Work out the finished part from the listing and answer in its coordinate system (mm). Round coordinates to 2 decimals unless told otherwise and drop trailing zeros. Loops run counter-clockwise (first coordinate to the right, second up) from the corner with the lowest first, then second, coordinate; pieces in that order, holes last. Notation, with made-up numbers: (-31, -18.75) -> (23, -18.75) arc R8 cw to (23, -14.75) -> close; hole circle Ø10 at (43.5, 28.5). An arc over 180 degrees is marked (long way). Use one line per item in the form item = value.
Autodesk Inventor part; units mm, degrees
ref_plane "YZ Plane" through (0, 0, 0) normal (1, 0, 0) x (0, 1, 0)
ref_plane "XZ Plane" through (0, 0, 0) normal (0, 1, 0) x (-1, 0, 0)
ref_plane "XY Plane" through (0, 0, 0) normal (0, 0, 1) x (1, 0, 0)
sketch "Sketch1" plane through (0, 0, 0) normal (0, 0, 1) x (1, 0, 0)
  circle A0 centre (0, 0) radius 10
  dimension "d0" = 20
extrude "Extrusion1" add sketch "Sketch1" along normal blind 5
sketch "Sketch2" plane through (0, 0, 5) normal (0, 0, 1) x (1, 0, 0)
  circle A0 centre (0, 0) radius 8.5
  dimension "d3" = 17
extrude "Extrusion2" add sketch "Sketch2" along normal blind 2.5
sketch "Sketch3" plane through (0, 0, 7.5) normal (0, 0, 1) x (1, 0, 0)
  circle A0 centre (0, 0) radius 9.9761
extrude "Extrusion3" add sketch "Sketch3" along normal blind 20
sketch "Sketch4" plane through (0, 0, 27.5) normal (0, 0, 1) x (1, 0, 0)
  circle A0 centre (0, 0) radius 8.5
extrude "Extrusion4" add sketch "Sketch4" along normal blind 2.5
sketch "Sketch5" plane through (0, 0, 30) normal (0, 0, 1) x (1, 0, 0)
  circle A0 centre (0, 0) radius 9.9761
extrude "Extrusion5" add sketch "Sketch5" along normal blind 5
sketch "Sketch6" plane through (0, 0, 35) normal (0, 0, 1) x (1, 0, 0)
  line L0 (-13.1636, 0) -> (14.8956, 0)
  line L1 (14.8956, 0) -> (14.8956, -10.45)
  line L2 (14.8956, -10.45) -> (-13.1636, -10.45)
  line L3 (-13.1636, -10.45) -> (-13.1636, 0)
  point P0 (0, 0)
extrude "Extrusion6" cut sketch "Sketch6" against normal blind 35
properties part number "Top Pully"
(1) Find section A-A, the plane x = 0. Write down the section's boundary in (y, z).
Completed:
outline = (0, 0) -> (10, 0) -> (10, 5) -> (8.5, 5) -> (8.5, 7.5) -> (9.98, 7.5) -> (9.98, 27.5) -> (8.5, 27.5) -> (8.5, 30) -> (9.98, 30) -> (9.98, 35) -> (0, 35) -> close
(2) Find section D-D, the plane x = -2.25. Write down the section's boundary in (y, z).
Completed:
outline = (0, 0) -> (9.74, 0) -> (9.74, 5) -> (8.2, 5) -> (8.2, 7.5) -> (9.72, 7.5) -> (9.72, 27.5) -> (8.2, 27.5) -> (8.2, 30) -> (9.72, 30) -> (9.72, 35) -> (0, 35) -> close
(3) For a pull along Z with two mould halves and no side action, classify faces 1 (the flat face through (0, 4, 35)), 2 (the cylindrical face through (-0.219, 9.974, 17.36)), 3 (the flat face through (-1, 9, 30)) as +Z half, -Z half, draft (parallel to the pull), parting line (faces both ways), or undercut.
Completed:
face_1 = +Z half
face_2 = draft
face_3 = undercut
(4) Consider L1, parallel to Z at x = 8.5, y = 1.75; L2, parallel to Y at x = 5.25, z = 8; L3, parallel to X at y = 6.25, z = 28. Determine where each line is inside the solid, lowest interval first.
Completed:
L1 = 0 to 5, 7.5 to 27.5, 30 to 35
L2 = 0 to 8.48
L3 = -5.76 to 5.76
(5) Find section B-B, the plane z = 16. Write down the section's boundary in (x, y), then the cut area to 3 significant figures.
Completed:
outline = (-9.98, 0) -> (9.98, 0) arc R9.98 ccw to start
area = 156 mm2
(6) Find section C-C, the plane y = 4. Write down the section's boundary in (x, z), then the cut area to 3 significant figures.
Completed:
outline = (-9.17, 0) -> (9.17, 0) -> (9.17, 5) -> (7.5, 5) -> (7.5, 7.5) -> (9.14, 7.5) -> (9.14, 27.5) -> (7.5, 27.5) -> (7.5, 30) -> (9.14, 30) -> (9.14, 35) -> (-9.14, 35) -> (-9.14, 30) -> (-7.5, 30) -> (-7.5, 27.5) -> (-9.14, 27.5) -> (-9.14, 7.5) -> (-7.5, 7.5) -> (-7.5, 5) -> (-9.17, 5) -> close
area = 624 mm2
(7) Given P1, Ø6, axis at y = 2, z = 14.5, coming from the +X side; P2, Ø1.5, axis at y = 4, z = 26, coming from the -X side; P3, Ø1, axis at y = 8, z = 13.5, coming from the -X side; P4, Ø2, axis at x = -1.5, y = 2.5, coming from the -Z side, each flat-ended and moving along its own axis, determine where each tip first touches the part or whether it passes through.
Completed:
P1 = 9.98
P2 = -9.43
P3 = -6.58
P4 = 0
